Drawing for the job (mm, zero at the part's lowest x, y, z). A direction names the side the tool comes from. Give positions to 0.01 mm unless a question says otherwise; leave off trailing zeros. Order: outer loops, then holes, each group sorted by start corner. A loop starts at its lowest first (then second) coordinate and runs counter-clockwise, first axis right, second up. Notation, with made-up numbers: (-31.75, 63) - (-22.75, 63) arc R13 cw to (-22.75, 76) - close; hole circle Ø9 at (-20.5, 82.5). An arc over 180 degrees is marked (long way). One line per item, written item: value.
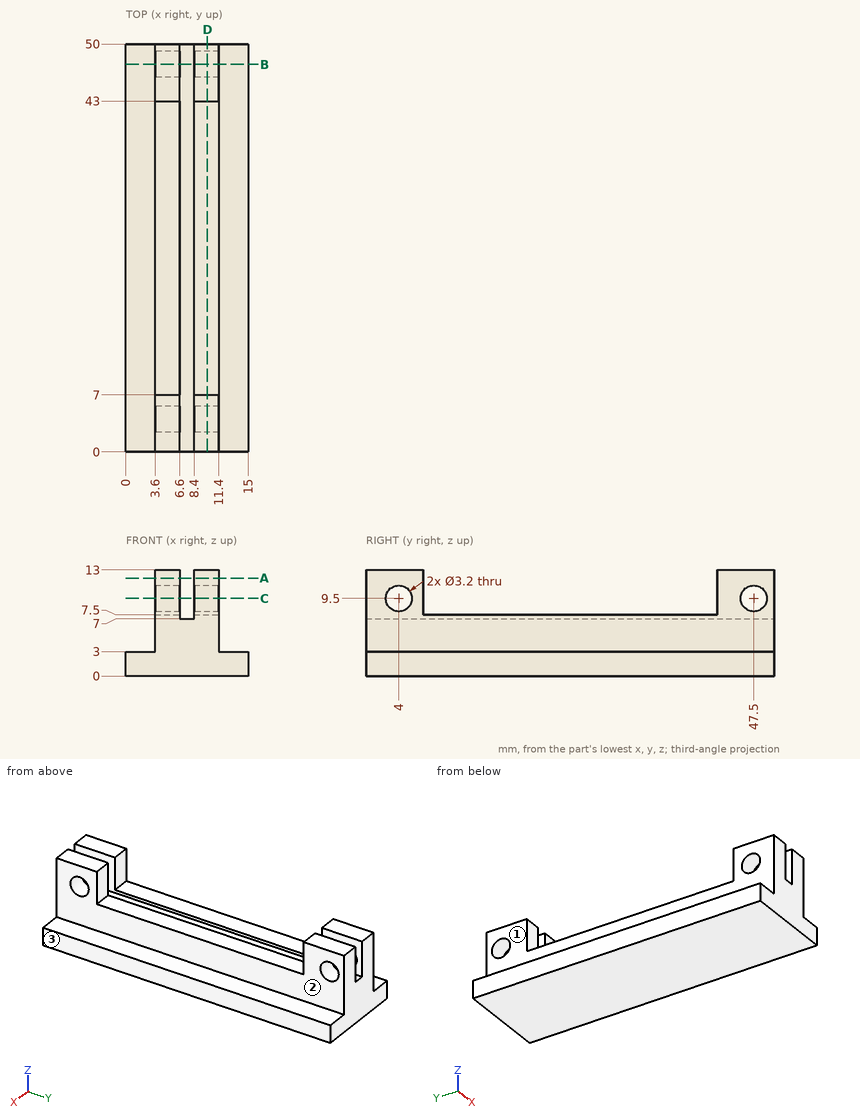
1) Cut at D-D, the plane x = 10. Give the cut face in (y, z), then the cut area to 3 significant figures.
Outcome:
outline: (0, 0) - (50, 0) - (50, 13) - (43, 13) - (43, 7.5) - (7, 7.5) - (7, 13) - (0, 13) - close; hole circle Ø3.2 at (4, 9.5); hole circle Ø3.2 at (47.5, 9.5)
area: 436 mm^2
2) Pin check, flat tips, straight feed: pin 1 (1.1 mm diameter, centred on x = 13, y = 28.5, fed in from +Z); pin 2 (4 mm diameter, centred on y = 4, z = 9.5, fed in from +X); pin 3 (1 mm diameter, centred on x = 8.5, z = 1.5, fed in from -Y); pin 4 (0.9 mm diameter, centred on x = 9, y = 20.5, fed in from +Z). Stop position of each tip, or through.
Outcome:
pin 1: stops at z = 3
pin 2: stops at x = 11.4
pin 3: stops at y = 0
pin 4: stops at z = 7.5
3) Cut at B-B, the plane y = 47.5. Give the cut face in (x, z), then the cut area to 3 significant figures.
Outcome:
outline: (0, 0) - (15, 0) - (15, 3) - (11.4, 3) - (11.4, 7.9) - (8.4, 7.9) - (8.4, 7) - (6.6, 7) - (6.6, 7.9) - (3.6, 7.9) - (3.6, 3) - (0, 3) - close; (3.6, 11.1) - (6.6, 11.1) - (6.6, 13) - (3.6, 13) - close; (8.4, 11.1) - (11.4, 11.1) - (11.4, 13) - (8.4, 13) - close
area: 93.0 mm^2
4) Which spindle directions (+Z, -Z, +X, -X, +Y, -Y) get a long thin tool onto all of the face, cutting with end or side? Do the marked faces 1, 2 and 3. Say none if no direction does.
Outcome:
face 1: +Z, -X, +Y, -Y
face 2: +Z, +X, +Y, -Y
face 3: +Z, -Z, +X, +Y, -Y
5) Drill centre lines: line 1 along Y through (x, z) = (5.55, 9.5); line 2 along X through (y, z) = (45, 8.75); line 3 along Y through (x, z) = (10.5, 8.5). Where is each one in solid material? Low to high. Write a range as from..to.
Outcome:
line 1: y = 0..2.4, 5.6..7, 43..45.9, 49.1..50
line 2: x = 3.6..6.6, 8.4..11.4
line 3: y = 0..2.75, 5.25..7, 43..46.25, 48.75..50
6) Cut at A-A, the plane z = 12. Give the cut face in (x, y).
Outcome:
outline: (3.6, 0) - (6.6, 0) - (6.6, 7) - (3.6, 7) - close; (3.6, 43) - (6.6, 43) - (6.6, 50) - (3.6, 50) - close; (8.4, 0) - (11.4, 0) - (11.4, 7) - (8.4, 7) - close; (8.4, 43) - (11.4, 43) - (11.4, 50) - (8.4, 50) - close
7) Cut at C-C, the plane z = 9.5. Give the number of separate pieces and of enclosed holes in the cut face, then the cut area to 3 significant figures.
Outcome:
separate pieces: 8
enclosed holes: 0
area: 45.6 mm^2
